from build123d import *

# Parameters (mm, degrees)
SKETCH_1_R               = 28.35
EXTRUDE_1_DEPTH          = 5
SKETCH_2_R               = 16
EXTRUDE_2_DEPTH          = 10
SKETCH_3_R               = 4
CUT_EXTRUDE_1_DEPTH      = 43.807067174
M5X0_8_1_D               = 4.2
PATTERN_CIRCULAR_1_COUNT = 6
SKETCH_11_W              = 2.1
SKETCH_11_H              = 16.001
PATTERN_CIRCULAR_2_COUNT = 2
PATTERN_CIRCULAR_2_ANGLE = 90
BOSS_EXTRUDE1_DEPTH      = 15


with BuildPart() as part:
    # 草圖1 → 填料-伸長1 (new body)
    with BuildSketch(Plane.XY):
        Circle(SKETCH_1_R)
    extrude(amount=EXTRUDE_1_DEPTH)

    # 草圖2 → 填料-伸長2 (add)
    with BuildSketch(Plane.XY.offset(5)):
        Circle(SKETCH_2_R)
    extrude(amount=EXTRUDE_2_DEPTH)

    # 草圖3 → 除料-伸長1 (cut, through all)
    with BuildSketch(Plane.XY.offset(15)):
        Circle(SKETCH_3_R)
    extrude(amount=-CUT_EXTRUDE_1_DEPTH, mode=Mode.SUBTRACT)

    # M5x0.8 螺紋孔1 (through all)
    with Locations(Plane(origin=(0, 23.75, 5), x_dir=(1, 0, 0), z_dir=(0, 0, 1))):
        with Locations((0, 0)):
            m5x0_8_1 = Hole(M5X0_8_1_D / 2)

    # 環狀複製排列1: M5x0.8 螺紋孔1 ×6 about axis
    pattern_circular_1_axis = Axis((0, 0, 0), (0, 0, 1))
    for i in range(1, PATTERN_CIRCULAR_1_COUNT):
        add(m5x0_8_1.rotate(pattern_circular_1_axis, i * 360 / PATTERN_CIRCULAR_1_COUNT), mode=Mode.SUBTRACT)

    # 草圖11 → M5x0.8 螺紋孔2 (revolve, cut)
    with BuildSketch(Plane(origin=(0, 0, 9), x_dir=(0, 0, 1), z_dir=(0, 1, 0))):
        with Locations((1.05, 8.0005)):
            Rectangle(SKETCH_11_W, SKETCH_11_H)
    m5x0_8_2 = revolve(axis=Axis((-6.35, 0, 9), (1, 0, 0)), mode=Mode.SUBTRACT)

    # 環狀複製排列2: M5x0.8 螺紋孔2 ×2 about axis
    pattern_circular_2_axis = Axis((0, 0, 15), (0, 0, 1))
    for i in range(1, PATTERN_CIRCULAR_2_COUNT):
        add(m5x0_8_2.rotate(pattern_circular_2_axis, i * PATTERN_CIRCULAR_2_ANGLE / (PATTERN_CIRCULAR_2_COUNT - 1)), mode=Mode.SUBTRACT)

    # Sketch1 → Boss-Extrude1 (add)
    with BuildSketch(Plane.XY.offset(15)):
        with BuildLine():
            ThreePointArc((4, 0), (1.414213562, 3.741657387), (-3, 2.645751311))
            Line((-3, 2.645751311), (-3, -2.645751311))
            ThreePointArc((-3, -2.645751311), (1.414213562, -3.741657387), (4, 0))
        make_face()
        with BuildLine():
            Line((-3, -2.645751311), (-3, 2.645751311))
            ThreePointArc((-3, 2.645751311), (-3.999997422, 0.0045417), (-3.006000366, -2.638931943))
            ThreePointArc((-3.006000366, -2.638931943), (-3.003002119, -2.64234333), (-3, -2.645751311))
        make_face()
    extrude(amount=BOSS_EXTRUDE1_DEPTH)


with BuildPart() as boss_extrude1_kept_piece:
    # of the separate pieces the step leaves, the one the design keeps (boss_extrude1_pieces_kept)
    add(part.part.solids().sort_by_distance((28.35, 0, 0))[0])


solid = boss_extrude1_kept_piece.part
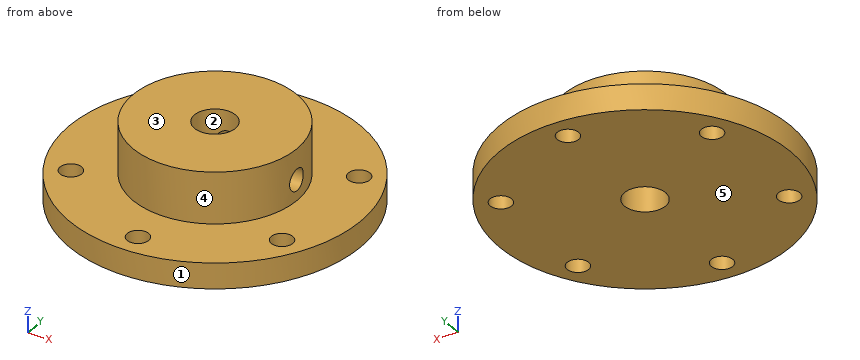
Model file for the job. Use its own axes, mm. Face numbers are marked on the shaded views. A direction names the side the tool comes from. Give positions to 0.01 mm unless a question says otherwise; leave off trailing zeros. Write each loop counter-clockwise with the first axis right and the second up, starting at its lowest first coordinate (ties: lowest second). Pieces come first, ordered by that corner, then holes. Notation, with made-up numbers: (3, -35) -> (23, -35) arc R13 cw to (23, -19) -> close; hole circle Ø10 at (14.5, -33.5). An arc over 180 degrees is marked (long way). Write item = value, one per line.
(1) Slice it at B-B, the plane z = 9.25. Give the cut face in (x, y), then the cut area to 3 significant figures.
Determined:
outline = (-2.09, 3.41) -> (-2.09, 15.86) arc R16 ccw (long way) to (15.86, -2.09) -> (3.41, -2.09) arc R4 cw (long way) to start; (2.09, 3.41) arc R4 cw to (3.41, 2.09) -> (15.86, 2.09) arc R16 ccw to (2.09, 15.86) -> close
area = 653 mm2
(2) Slice it at D-D, the plane y = -23.75. Give the cut face in (x, z).
Determined:
outline = (-15.48, 0) -> (-2.1, 0) -> (-2.1, 5) -> (-15.48, 5) -> close; (2.1, 0) -> (15.48, 0) -> (15.48, 5) -> (2.1, 5) -> close
(3) Slice it at A-A, the plane y = 0. Give the cut face in (x, z), then the cut area to 3 significant figures.
Determined:
outline = (-28.35, 0) -> (-4, 0) -> (-4, 15) -> (-16, 15) -> (-16, 5) -> (-28.35, 5) -> close; (4, 0) -> (28.35, 0) -> (28.35, 5) -> (16, 5) -> (16, 6.9) -> (4, 6.9) -> close; (4, 11.1) -> (16, 11.1) -> (16, 15) -> (4, 15) -> close
area = 433 mm2
(4) Tool access for the marked faces 4 and 5: list every direction of +Z, -Z, +X, -X, +Y, -Y with a clear straight run to the whole face (end or side of a thin tool).
Determined:
face_4 = +Z
face_5 = -Z, +X, -X, +Y, -Y
(5) Flat gauge pins, fed straight in: P1, Ø1.5, axis at x = -17.5, y = -6, coming from the -Z side; P2, Ø2, axis at y = 0.5, z = 7, coming from the +X side; P3, Ø5, axis at x = 4.5, z = 5, coming from the -Y side; P4, Ø4, axis at y = 0, z = 9, coming from the -X side. Where does each tip first touch, or does it go through?
Determined:
P1 = 0
P2 = 16
P3 = -28.28
P4 = -16
(6) Slice it at C-C, the plane x = 0. Give the cut face in (y, z).
Determined:
outline = (-28.35, 0) -> (-25.85, 0) -> (-25.85, 5) -> (-28.35, 5) -> close; (-21.65, 0) -> (-4, 0) -> (-4, 15) -> (-16, 15) -> (-16, 5) -> (-21.65, 5) -> close; (4, 0) -> (21.65, 0) -> (21.65, 5) -> (16, 5) -> (16, 6.9) -> (4, 6.9) -> close; (4, 11.1) -> (16, 11.1) -> (16, 15) -> (4, 15) -> close; (25.85, 0) -> (28.35, 0) -> (28.35, 5) -> (25.85, 5) -> close
(7) Probe line 1 along Y through (x, z) = (0, 1.1); line 2 along Z through (x, y) = (12, 23.5); line 3 along X through (y, z) = (-22.5, 4). List the from-to ranges inside material, lowest first.
Determined:
line_1 = -28.35 to -25.85, -21.65 to -4, 4 to 21.65, 25.85 to 28.35
line_2 = 0 to 5
line_3 = -17.25 to -1.69, 1.69 to 17.25
(8) Mould opens along Y. For the marked faces 1, 2 and 3 say: released by +Y, released by -Y, zero draft, split by the parting line, or undercut.
Determined:
face_1 = split by the parting line
face_2 = undercut
face_3 = zero draft
